Geometry check sheet. Reference: the model listing, model coordinates, mm. Face numbers are marked on the shaded views. A direction names the side the tool comes from. Coordinates: 2 decimals unless noted, no trailing zeros. Write each loop counter-clockwise with the first axis right and the second up, starting at its lowest first coordinate (ties: lowest second). Pieces come first, ordered by that corner, then holes. Notation, with made-up numbers: (63.5, 45.5) - (122.5, 45.5) arc R30 ccw to (122.5, 81.5) - close; hole circle Ø9 at (-11.75, -23.5). An arc over 180 degrees is marked (long way). Answer as a JSON object with one key per item and string values. Group by question number.
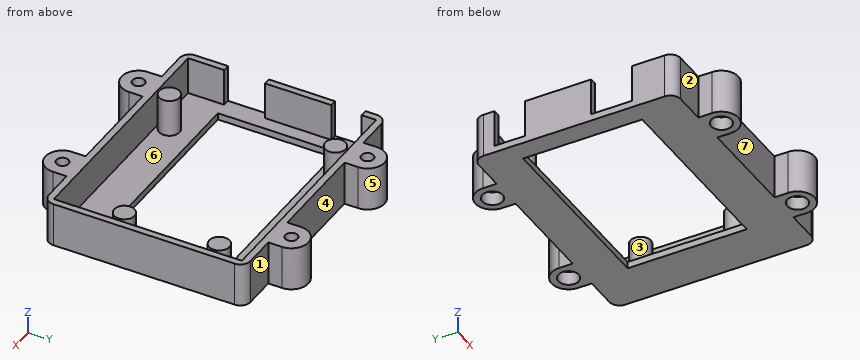
from build123d import *

# Parameters (mm, degrees)
SKETCH_R        = 1.8
PAD_DEPTH       = 13
SKETCH001_W     = 70.6
SKETCH001_H     = 55.3
POCKET_DEPTH    = 11
SKETCH002_R     = 3
PAD001_DEPTH    = 11
SKETCH004_R     = 3
POCKET001_DEPTH = 4
SKETCH005_R     = 3
POCKET002_DEPTH = 4
SKETCH007_W     = 12
SKETCH007_H     = 11
SKETCH007_W_2   = 8.9
POCKET003_DEPTH = 2
SKETCH008_W     = 55
SKETCH008_H     = 35
POCKET004_DEPTH = 5


with BuildPart() as part:
    # Sketch → Pad (new body)
    with BuildSketch(Plane.XY):
        with BuildLine():
            ThreePointArc((-3, 0), (-2.12132, -2.12132), (0, -3))
            Line((0, -3), (9.3, -3))
            Line((9.3, -3), (9.3, -7))
            ThreePointArc((9.3, -7), (14.3, -12), (19.3, -7))
            Line((19.3, -7), (19.3, -3))
            Line((19.3, -3), (49.3, -3))
            Line((49.3, -3), (49.3, -7))
            ThreePointArc((49.3, -7), (54.3, -12), (59.3, -7))
            Line((59.3, -7), (59.3, -3))
            Line((59.3, -3), (68.6, -3))
            ThreePointArc((68.6, -3), (70.72132, -2.12132), (71.6, 0))
            Line((71.6, 0), (71.6, 53.3))
            ThreePointArc((71.6, 53.3), (70.72132, 55.42132), (68.6, 56.3))
            Line((59.3, 56.3), (68.6, 56.3))
            Line((59.3, 60.3), (59.3, 56.3))
            ThreePointArc((59.3, 60.3), (54.3, 65.3), (49.3, 60.3))
            Line((49.3, 56.3), (49.3, 60.3))
            Line((19.3, 56.3), (49.3, 56.3))
            Line((19.3, 60.3), (19.3, 56.3))
            ThreePointArc((19.3, 60.3), (14.3, 65.3), (9.3, 60.3))
            Line((9.3, 56.3), (9.3, 60.3))
            Line((0, 56.3), (9.3, 56.3))
            ThreePointArc((0, 56.3), (-2.12132, 55.42132), (-3, 53.3))
            Line((-3, 53.3), (-3, 0))
        make_face()
        with Locations((14.3, -7)):
            Circle(SKETCH_R, mode=Mode.SUBTRACT)
        with Locations((54.3, -7)):
            Circle(SKETCH_R, mode=Mode.SUBTRACT)
        with Locations((54.3, 60.3)):
            Circle(SKETCH_R, mode=Mode.SUBTRACT)
        with Locations((14.3, 60.3)):
            Circle(SKETCH_R, mode=Mode.SUBTRACT)
    extrude(amount=PAD_DEPTH)

    # Sketch001 → Pocket (cut)
    with BuildSketch(Plane.XY.offset(13)):
        with Locations((34.3, 26.65)):
            Rectangle(SKETCH001_W, SKETCH001_H)
    extrude(amount=-POCKET_DEPTH, mode=Mode.SUBTRACT)

    # Sketch002 → Pad001 (new body)
    with BuildSketch(Plane.XY.offset(2)):
        with Locations((14, 50.7)):
            Circle(SKETCH002_R)
        with Locations((15.1, 2.5)):
            Circle(SKETCH002_R)
        with Locations((65.9, 45.6)):
            Circle(SKETCH002_R)
        with Locations((65.9, 17.7)):
            Circle(SKETCH002_R)
    extrude(amount=PAD001_DEPTH)

    # Sketch004 → Pocket001 (cut)
    with BuildSketch(Plane(origin=(0, 0, 0), x_dir=(1, 0, 0), z_dir=(0, 0, -1))):
        with Locations((54.3, 7)):
            Circle(SKETCH004_R)
        with Locations((14.3, 7)):
            Circle(SKETCH004_R)
    extrude(amount=-POCKET001_DEPTH, mode=Mode.SUBTRACT)

    # Sketch005 → Pocket002 (cut)
    with BuildSketch(Plane(origin=(0, 0, 0), x_dir=(1, 0, 0), z_dir=(0, 0, -1))):
        with Locations((54.3, -60.3)):
            Circle(SKETCH005_R)
        with Locations((14.3, -60.3)):
            Circle(SKETCH005_R)
    extrude(amount=-POCKET002_DEPTH, mode=Mode.SUBTRACT)

    # Sketch007 → Pocket003 (cut)
    with BuildSketch(Plane(origin=(-3, 0, 0), x_dir=(0, -1, 0), z_dir=(-1, 0, 0))):
        with Locations((-15.6, 7.5)):
            Rectangle(SKETCH007_W, SKETCH007_H)
        with Locations((-45.55, 7.5)):
            Rectangle(SKETCH007_W_2, SKETCH007_H)
    extrude(amount=-POCKET003_DEPTH, mode=Mode.SUBTRACT)

    # Sketch008 → Pocket004 (cut)
    with BuildSketch(Plane(origin=(0, 0, 0), x_dir=(1, 0, 0), z_dir=(0, 0, -1))):
        with Locations((30.5, -27.5)):
            Rectangle(SKETCH008_W, SKETCH008_H)
    extrude(amount=-POCKET004_DEPTH, mode=Mode.SUBTRACT)


solid = part.part
(1) Draft check along Y on the marked faces 5, 6 and 7. Enter one of: +Y half, -Y half, draft (parallel to the pull), parting line (faces both ways), or undercut.
(2) Section check A-A (x = 54.3). Record the cut outline in (y, z).
(3) Section check D-D (x = 4). Record the cut outline in (y, z).
(4) Set-up check for the marked faces 1, 2, 3 and 4: record each of +Z, -Z, +X, -X, +Y, -Y from which the full face is reachable in a straight line by a thin tool's end or side.
(5) Section check C-C (z = 6.5). Count the separate pieces of the cut face and the enclosed holes in it, and give its area (3 significant figures).
(6) Material ranges on L1, parallel to X at y = 60.3, z = 0.8; L2, parallel to X at y = -7, z = 10.25; L3, parallel to Y at x = 27, z = 1.5, recorded low to high. Write a range as [from, to].
(7) Section check B-B (y = 34). Record the cut outline in (x, z), and give its area (3 significant figures).
(8) Gauge pin test, flat ends, axial feed: pin 1 (5 mm diameter, centred on x = 10, z = 3, fed in from +Y); pin 2 (3 mm diameter, centred on x = 3.5, z = 9.5, fed in from -Y); pin 3 (4.5 mm diameter, centred on y = -5.5, z = 6.5, fed in from -X). Record the tip position at first contact, or that the pin passes through.
Conclusion:
{
 "1": {"face 5": "+Y half", "face 6": "undercut", "face 7": "-Y half"},
 "2": {"outline": "(-12, 0) - (-10, 0) - (-10, 4) - (-8.8, 4) - (-8.8, 13) - (-12, 13) - close; (-5.2, 4) - (-4, 4) - (-4, 0) - (10, 0) - (10, 2) - (-1, 2) - (-1, 13) - (-5.2, 13) - close; (45, 0) - (57.3, 0) - (57.3, 4) - (58.5, 4) - (58.5, 13) - (54.3, 13) - (54.3, 2) - (45, 2) - close; (62.1, 4) - (63.3, 4) - (63.3, 0) - (65.3, 0) - (65.3, 13) - (62.1, 13) - close"},
 "3": {"outline": "(-3, 0) - (10, 0) - (10, 2) - (-1, 2) - (-1, 13) - (-3, 13) - close; (45, 0) - (56.3, 0) - (56.3, 13) - (54.3, 13) - (54.3, 2) - (45, 2) - close"},
 "4": {"face 1": "+Z, -Z, +X, +Y", "face 2": "+Z, -Z, -X, -Y", "face 3": "+Z", "face 4": "+Z, -Z, +Y"},
 "5": {"separate pieces": "6", "enclosed holes": "4", "area": "860 mm^2"},
 "6": {"L1": "x = [9.3, 11.3], [17.3, 19.3], [49.3, 51.3], [57.3, 59.3]", "L2": "x = [9.3, 12.5], [16.1, 19.3], [49.3, 52.5], [56.1, 59.3]", "L3": "y = [-3, 10], [45, 56.3]"},
 "7": {"outline": "(-3, 0) - (3, 0) - (3, 2) - (-1, 2) - (-1, 13) - (-3, 13) - close; (58, 0) - (71.6, 0) - (71.6, 13) - (69.6, 13) - (69.6, 2) - (58, 2) - close", "area": "83.2 mm^2"},
 "8": {"pin 1": "stops at y = 64.96", "pin 2": "stops at y = -3", "pin 3": "stops at x = 9.3"}
}
